Read the model definition and answer for the solid it produces. Units are mm, in the model's axes. A direction names the side the tool comes from. Give positions to 0.01 mm unless a question says otherwise; leave off trailing zeros. Write each loop counter-clockwise with the first axis right and the second up, starting at its lowest first coordinate (ties: lowest second). Pieces come first, ordered by that corner, then holes. Notation, with made-up numbers: (64, 57.25) -> (82, 57.25) arc R17 cw to (82, 69.25) -> close; hole circle Ø9 at (30.5, 36). An arc over 180 degrees is marked (long way). Use a Markdown table: item, result.
from build123d import *

# Parameters (mm, degrees)
SKIZZE1_W                       = 392.409898916
SKIZZE1_H                       = 368.579338253
AUFSATZ_LINEAR_AUSTRAGEN1_DEPTH = 3


with BuildPart() as part:
    # Skizze1 → Aufsatz-Linear austragen1 (new body)
    with BuildSketch(Plane.XY):
        with Locations((3.931385317, -27.213089131)):
            Rectangle(SKIZZE1_W, SKIZZE1_H)
        with BuildLine():
            ThreePointArc((29.936886891, 72.802324452), (-7.660783232, 74.856809504), (-45, 70))
            ThreePointArc((-45, 70), (-50, 0), (-45, -70))
            ThreePointArc((-45, -70), (-7.660783232, -74.856809504), (29.936886891, -72.802324452))
            ThreePointArc((29.936886891, -72.802324452), (41.39751926, -66.915583853), (46.889917221, -55.260826292))
            ThreePointArc((46.889917221, -55.260826292), (50, 0), (46.889917221, 55.260826292))
            ThreePointArc((46.889917221, 55.260826292), (41.39751926, 66.915583853), (29.936886891, 72.802324452))
        make_face(mode=Mode.SUBTRACT)
    extrude(amount=AUFSATZ_LINEAR_AUSTRAGEN1_DEPTH)


solid = part.part
Item 1: For a pull along X with two mould halves and no side action, classify faces 3 (the face through (41.525, 66.783, 1.479)), 4 (the face through (45, -66, 3)) as +X half, -X half, draft (parallel to the pull), parting line (faces both ways), or undercut.
Return value:
| item | result |
|---|---|
| face 3 | undercut |
| face 4 | draft |
Item 2: Straight lines are drawn through the part: line 1 along X through (y, z) = (7.5, 1.85); line 2 along Y through (x, z) = (-3.5, 2.2); line 3 along X through (y, z) = (-15.5, 2.1). For each, find the intervals that lie inside material, in ascending order. Write a range as [from, to].
Return value:
| item | result |
|---|---|
| line 1 | [-192.27, -49.94], [49.94, 200.14] |
| line 2 | [-211.5, -74.97], [74.97, 157.08] |
| line 3 | [-192.27, -49.76], [49.76, 200.14] |
Item 3: A cutting plane is placed at A-A (z = 2.3). Give the vertices of the cut face in (x, y).
Return value:
| item | result |
|---|---|
| outline | (-192.27, -211.5) -> (200.14, -211.5) -> (200.14, 157.08) -> (-192.27, 157.08) -> close; hole (-45, -70) arc R205 ccw to (29.94, -72.8) arc R20 ccw to (46.89, -55.26) arc R492.5 ccw to (46.89, 55.26) arc R20 ccw to (29.94, 72.8) arc R205 ccw to (-45, 70) arc R492.5 ccw to start |
Item 4: A cutting plane is placed at B-B (y = -40.5). Give the vertices of the cut face in (x, z), then the cut area to 3 significant figures.
Return value:
| item | result |
|---|---|
| outline | (-192.27, 0) -> (-48.33, 0) -> (-48.33, 3) -> (-192.27, 3) -> close; (48.33, 0) -> (200.14, 0) -> (200.14, 3) -> (48.33, 3) -> close |
| area | 887 mm^2 |
Item 5: A tool of negligible diameter and unlimited length cuts with its end or side. For faces 1 (the face through (41.269, -67.047, 1.479)), 2 (the face through (45, -66, 0)), from which of +Z, -Z, +X, -X, +Y, -Y can it reach the whole face along a straight path? Write none if from no direction.
Return value:
| item | result |
|---|---|
| face 1 | +Z, -Z |
| face 2 | -Z, +X, -X, +Y, -Y |
Item 6: A cutting plane is placed at C-C (x = -25). Give the vertices of the cut face in (y, z), then the cut area to 3 significant figures.
Return value:
| item | result |
|---|---|
| outline | (-211.5, 0) -> (-73.47, 0) -> (-73.47, 3) -> (-211.5, 3) -> close; (73.47, 0) -> (157.08, 0) -> (157.08, 3) -> (73.47, 3) -> close |
| area | 665 mm^2 |
